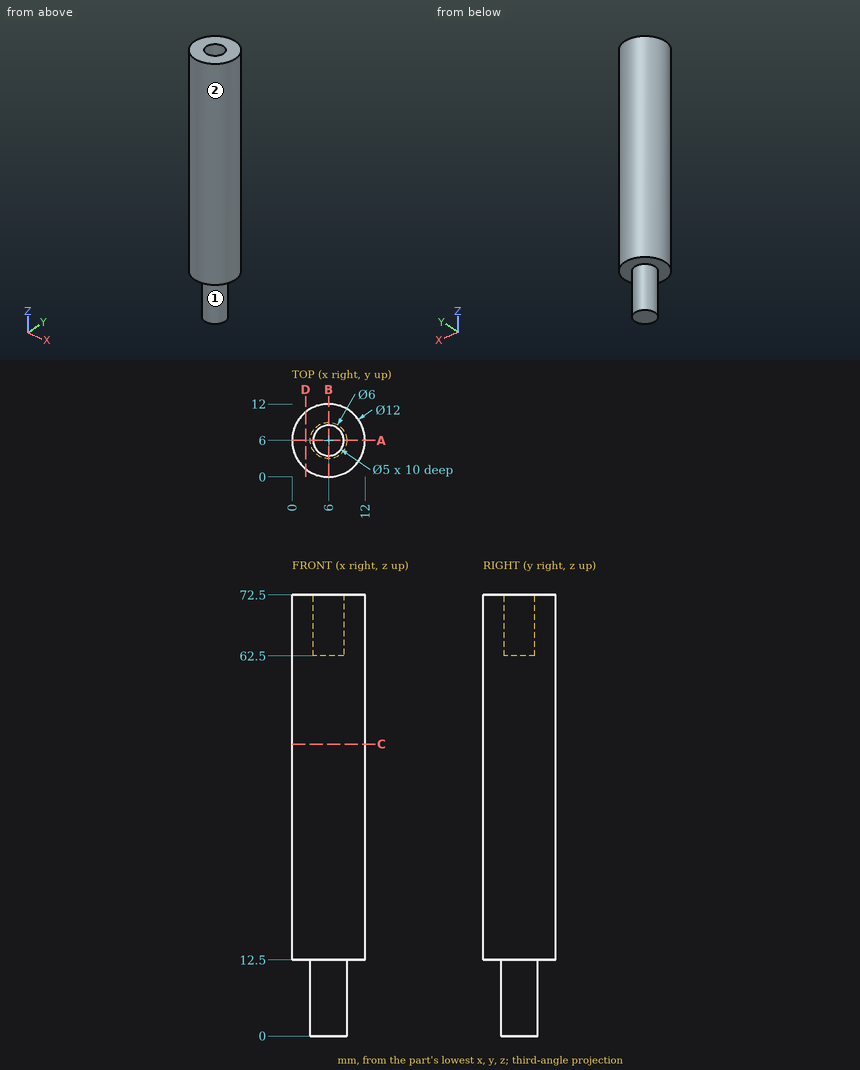
Geometry: see drawing. Coordinates: mm, zero at the bounding-box minimum. A direction names the side the tool comes from. Give positions to 0.01 mm unless a question says otherwise; leave off trailing zeros. Write each loop counter-clockwise with the first axis right and the second up, starting at its lowest first coordinate (ties: lowest second). Pieces come first, ordered by that corner, then holes. Notation, with made-up numbers: M 7.25,83.25 L 57.25,83.25 A21 ccw 57.25,120.25 Z; hole C 53.25,19.25 d7. An arc over 180 degrees is marked long. Return JSON: item names as keys, results as strings. Group by question number.
1) First-contact query: pin 1 Ø6 at (x, y) = (3.5, 6.5) entering from -Z; pin 2 Ø1.5 at (x, z) = (3, 18) entering from -Y; pin 3 Ø5 at (x, z) = (3, 47) entering from +Y; pin 4 Ø2 at (y, z) = (3.5, 46) entering from -X. Flat tips, straight axial feed; report the tip coordinate or a pass-through.
2) Set-up query: the marked faces 1 and 2. Return all of +Z, -Z, +X, -X, +Y, -Y with unobstructed straight access to the full face (end or side cutting, diameter ignored); none if empty.
3) Cut plane C-C, the plane z = 48. Output: boundary loops of the cut face in (x, y).
4) Cut plane D-D, the plane x = 2.25. Output: boundary loops of the cut face in (y, z), then the cut area to 3 significant figures.
5) Ray query, L1, parallel to Y at x = 6, z = 66.75; L2, parallel to Z at x = 5, y = 7.25; L3, parallel to Z at x = 8.75, y = 11. Return the intervals inside material, ascending.
6) Cut plane A-A, the plane y = 6. Output: boundary loops of the cut face in (x, z).
Data:
{
 "1": {"pin 1": "stops at z = 0", "pin 2": "stops at y = 0.44", "pin 3": "stops at y = 11.98", "pin 4": "stops at x = 0.19"},
 "2": {"face 1": "-Z", "face 2": "+Z, -Z"},
 "3": {"outline": "C 6,6 d12"},
 "4": {"outline": "M 1.32,12.5 L 10.68,12.5 L 10.68,72.5 L 1.32,72.5 Z", "area": "562 mm²"},
 "5": {"L1": "y = 0 to 3.5, 8.5 to 12", "L2": "z = 0 to 62.5", "L3": "z = 12.5 to 72.5"},
 "6": {"outline": "M 0,12.5 L 3,12.5 L 3,0 L 9,0 L 9,12.5 L 12,12.5 L 12,72.5 L 8.5,72.5 L 8.5,62.5 L 3.5,62.5 L 3.5,72.5 L 0,72.5 Z"}
}
